Source: CAD feature listing. Evaluate the final solid. Frame: model axes, mm. Face numbers are marked on the shaded views. A direction names the side the tool comes from. Round coordinates to 2 decimals unless told otherwise and drop trailing zeros. Loops run counter-clockwise (first coordinate to the right, second up) from the corner with the lowest first, then second, coordinate; pieces in that order, holes last. Notation, with made-up numbers: M 46.5,49 L 92.5,49 A20 ccw 92.5,88 Z; hole C 23.5,-17 d6. An arc over 180 degrees is marked long. One line per item, written item: value.
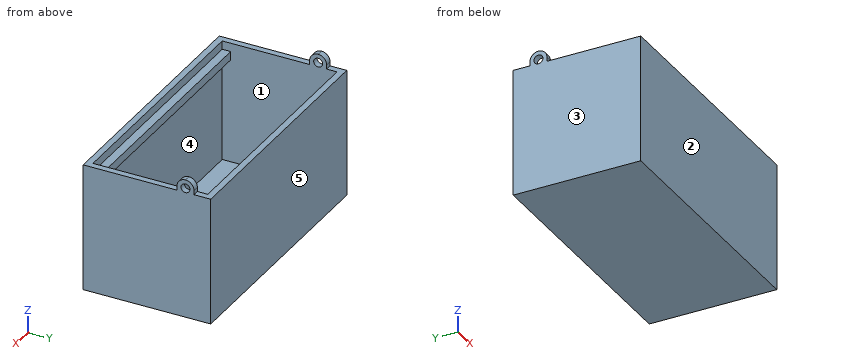
from build123d import *

# Parameters (mm, degrees)
F0_W      = 152.4
F0_H      = 76.2
F1_DEPTH  = 76.2
F2_T      = -3.81
F3_W      = 3.81
F3_H      = 10.16
F4_DEPTH  = 7.62
F5_R      = 2.667
F6_DEPTH  = 152.401
F7_R      = 5.07999
F8_W      = 144.78
F8_H      = 5.08
F9_DEPTH  = 5.08
F11_DEPTH = 144.78


# Not quite as in the source:
# - a fillet or chamfer is up to 0.001 mm smaller than in the source, because OpenCascade refuses the exact size


with BuildPart() as f1:
    # F0 (on Top) → F1 (new body)
    with BuildSketch(Plane.XY):
        Rectangle(F0_W, F0_H)
    extrude(amount=F1_DEPTH)

    # F2
    f2_openings = [f1.faces().sort_by_distance(p)[0] for p in [
        (0, 0, 76.2),
    ]]
    offset(amount=F2_T, openings=f2_openings)

    # F3 (on face) → F4 (join)
    with BuildSketch(Plane.XY.offset(76.2)):
        with Locations((-74.295, 23.0027831805)):
            Rectangle(F3_W, F3_H)
        with Locations((74.295, 23.0027831805)):
            Rectangle(F3_W, F3_H)
    extrude(amount=F4_DEPTH)

    # F5 (on face) → F6 (cut, through all)
    with BuildSketch(Plane.YZ.offset(76.2)):
        with Locations((23.0027831805, 78.74)):
            Circle(F5_R)
    extrude(amount=-F6_DEPTH, mode=Mode.SUBTRACT)

    # F7 (radius 5.08 in the source; OpenCascade refuses exactly that, so slightly less here)
    f7_edges = [f1.edges().sort_by_distance(p)[0] for p in [
        (74.295, 17.922783, 83.82),
        (74.295, 28.082783, 83.82),
        (-74.295, 28.082783, 83.82),
        (-74.295, 17.922783, 83.82),
    ]]
    fillet(f7_edges, radius=F7_R)

    # F8 (on face) → F9 (join)
    with BuildSketch(Plane(origin=(0, -34.29, 0), x_dir=(-1, 0, 0), z_dir=(0, 1, 0))):
        with Locations((0, 68.58)):
            Rectangle(F8_W, F8_H)
    extrude(amount=F9_DEPTH)

    # F10 (on face) → F11 (join)
    with BuildSketch(Plane.YZ.offset(-72.39)):
        Polygon((-34.29, 60.96), (-29.21, 66.04), (-34.29, 66.04), align=None)
    extrude(amount=F11_DEPTH)


solid = f1.part
1. Reachability of the marked faces 4 and 5 from +Z, -Z, +X, -X, +Y, -Y: full face, straight path, thin tool, end or side. Return the list, or none.
Report:
face 4: none
face 5: +Z, -Z, +X, -X, +Y
2. Ray query, line 1 (Y direction, x = 66, z = 16.5); line 2 (X direction, y = 21, z = 17.5); line 3 (Y direction, x = 62, z = 63.5). Return the intervals inside material, ascending. Write a range as [from, to].
Report:
line 1: y = [-38.1, -34.29], [34.29, 38.1]
line 2: x = [-76.2, -72.39], [72.39, 76.2]
line 3: y = [-38.1, -31.75], [34.29, 38.1]
3. Pull-direction query (X, two-part tool) for the marked faces 1, 2 and 3; classes: released by +X, released by -X, zero draft, split by the parting line, or undercut.
Report:
face 1: undercut
face 2: zero draft
face 3: released by -X
4. Section query A-A (z = 34). Return the cut outline in (x, y).
Report:
outline: M -76.2,-38.1 L 76.2,-38.1 L 76.2,38.1 L -76.2,38.1 Z; hole M -72.39,-34.29 L 72.39,-34.29 L 72.39,34.29 L -72.39,34.29 Z
5. Section query B-B (x = -57). Return the cut outline in (y, z).
Report:
outline: M -38.1,0 L 38.1,0 L 38.1,76.2 L 34.29,76.2 L 34.29,3.81 L -34.29,3.81 L -34.29,60.96 L -29.21,66.04 L -29.21,71.12 L -34.29,71.12 L -34.29,76.2 L -38.1,76.2 Z
6. Pin query (flat end, axial travel): pin 1 (8 mm diameter, centred on x = -24, y = 31, fed in from +Z); pin 2 (3 mm diameter, centred on x = 59.5, y = 19, fed in from -Z); pin 3 (2 mm diameter, centred on x = -74, z = 77.5, fed in from -Y); pin 4 (4 mm diameter, centred on x = 6, y = -12.5, fed in from +Z). Return the tip coordinate at first contact, or that it passes through.
Report:
pin 1: stops at z = 76.2
pin 2: stops at z = 0
pin 3: stops at y = 17.92
pin 4: stops at z = 3.81
7. Section query D-D (z = 69.5). Return the cut outline in (x, y), and give its area (3 significant figures).
Report:
outline: M -76.2,-38.1 L 76.2,-38.1 L 76.2,38.1 L -76.2,38.1 Z; hole M -72.39,-29.21 L 72.39,-29.21 L 72.39,34.29 L -72.39,34.29 Z
area: 2,420 mm2
8. Section query C-C (y = -26.5). Return the cut outline in (x, z).
Report:
outline: M -76.2,0 L 76.2,0 L 76.2,76.2 L 72.39,76.2 L 72.39,3.81 L -72.39,3.81 L -72.39,76.2 L -76.2,76.2 Z
